Source: CAD feature listing. Evaluate the final solid. Frame: model axes, mm. A direction names the side the tool comes from. Give positions to 0.01 mm unless a question says otherwise; leave off trailing zeros. Loops run counter-clockwise (first coordinate to the right, second up) from the corner with the lowest first, then second, coordinate; pieces in that order, holes last. Notation, with made-up numbers: (-39.5, 88.5) - (-15.5, 88.5) arc R22 ccw to (-15.5, 121.5) - close; hole circle Ø11 at (-9.5, 45.5). An arc over 180 degrees is marked (long way). Put each result on its own line as item: value.
Autodesk Inventor part; units mm, degrees
ref_plane "YZ Plane" through (0, 0, 0) normal (1, 0, 0) x (0, 1, 0)
ref_plane "XZ Plane" through (0, 0, 0) normal (0, 1, 0) x (-1, 0, 0)
ref_plane "XY Plane" through (0, 0, 0) normal (0, 0, 1) x (1, 0, 0)
sketch "Sketch1" plane through (0, 0, 0) normal (0, 0, 1) x (1, 0, 0)
  line L0 (-4, 10) -> (-4, 14)
  line L1 (0, 10) -> (-4, 10)
  line L2 (0, 14) -> (0, 10) construction
  line L3 (0, 14) -> (-4, 14)
  line L4 (-4, -16) -> (-4, 0)
  line L5 (0, -16) -> (-4, -16)
  line L6 (0, 0) -> (0, -16) construction
  line L7 (0, 0) -> (-4, 0)
  line L8 (0, 6.5) -> (0, 3.5)
  line L9 (0, 6.5) -> (12, 6.5)
  line L10 (12, 6.5) -> (12, 3.5)
  line L11 (12, 3.5) -> (0, 3.5)
  line L12 (0, 3.5) -> (0, 6.5)
  line L13 (0, 10) -> (0, 6.5)
  line L14 (0, 3.5) -> (0, 0)
  line L15 (4.8, 7.7) -> (7.2, 7.7)
  line L16 (7.2, 7.7) -> (7.2, 2.3)
  line L17 (7.2, 2.3) -> (4.8, 2.3)
  line L18 (4.8, 2.3) -> (4.8, 7.7)
  line L19 (11.3, -2.5) -> (23.3, -2.5)
  line L20 (23.3, -2.5) -> (23.3, -5.5)
  line L21 (23.3, -5.5) -> (11.3, -5.5)
  line L22 (11.3, -5.5) -> (11.3, -2.5)
  line L23 (16.1, -1.3) -> (18.5, -1.3)
  line L24 (18.5, -1.3) -> (18.5, -6.7)
  line L25 (18.5, -6.7) -> (16.1, -6.7)
  line L26 (16.1, -6.7) -> (16.1, -1.3)
  line L27 (0, 14) -> (27.3, 14)
  line L28 (27.3, 14) -> (27.3, 4)
  line L29 (27.3, 4) -> (23.3, 4)
  line L30 (23.3, 4) -> (23.3, -12)
  line L31 (23.3, -12) -> (27.3, -12)
  line L32 (27.3, -12) -> (27.3, -16)
  line L33 (27.3, -16) -> (0, -16)
  point P0 (7.2, 5)
  point P1 (12, 5)
  point P2 (6, 7.7)
  point P3 (6, 6.5)
  point P4 (16.1, -4)
  point P5 (11.3, -4)
  point P6 (17.3, -1.3)
  point P7 (17.3, -2.5)
  point P8 (23.3, -4)
  point P9 (23.3, -4)
  point P10 (4.8, 6.5)
  point P11 (7.2, 6.5)
  point P12 (7.2, 3.5)
  point P13 (4.8, 3.5)
  point P14 (18.5, -5.5)
  point P15 (16.1, -5.5)
  point P16 (16.1, -2.5)
  point P17 (18.5, -2.5)
  dimension "d0" = 12
  dimension "d1" = 3
  dimension "d2" = 5.4
  dimension "d3" = 2.4
  dimension "d4" = 12
  dimension "d5" = 3
  dimension "d6" = 2.4
  dimension "d7" = 5.4
  dimension "d8" = 4
  dimension "d10" = 10
  dimension "d11" = 23.3
  dimension "d12" = 4
extrude "Extrusion1" add sketch "Sketch1" along normal blind 4 contours L0 L3 L27 L28 L29 L30 L19 L24 L23 L26 L22 L21 L25 L31 L32 L33 L5 L4 L7 L14 L11 L18 L17 L16 L10 L9 L15 L13 L1
properties part number "Door_LimitSwitch_Holder_Side_1" material "MDF Medium Density Fiberboard"
1) Access query for faces 4 (the flat face through (12, -16, 2)), 5 (the flat face through (2, 3.5, 2)), 6 (the flat face through (21, -2.5, 2)), 7 (the flat face through (16.1, -6, 2)). Directions: +Z, -Z, +X, -X, +Y, -Y. A direction counts if a zero-diameter tool reaches every point of the face in a straight line with its end or side. Return the directions, or none.
Check result:
face 4: +Z, -Z, +X, -X, -Y
face 5: +Z, -Z, -X
face 6: +Z, -Z, +X
face 7: +Z, -Z
2) Mould query, pull axis X, two halves, no side actions, for faces 1 (the flat face through (-4, 12, 2)), 2 (the flat face through (18.5, -6, 2)), 3 (the flat face through (11, 14, 2)). Classes: pulls with the +X half, pulls with the -X half, needs draft (parallel to the pull), parting line crosses it, or undercut.
Check result:
face 1: pulls with the -X half
face 2: undercut
face 3: needs draft
3) Section query C-C, the plane y = -8.25. Output: boundary loops of the cut face in (x, z), plus the area to 3 significant figures.
Check result:
outline: (-4, 0) - (23.3, 0) - (23.3, 4) - (-4, 4) - close
area: 109 mm²
4) Pin query (flat end, axial travel): P1, Ø1.3, axis at y = -2, z = 2, coming from the +X side; P2, Ø0.6, axis at y = 7, z = 1.5, coming from the -X side; P3, Ø0.9, axis at y = -3.5, z = 2.5, coming from the +X side. Return the tip coordinate at first contact, or that it passes through.
Check result:
P1: x = 23.3
P2: x = 0
P3: x = 11.3
5) Section query A-A, the plane x = 12.5. Output: boundary loops of the cut face in (y, z), plus the area to 3 significant figures.
Check result:
outline: (-16, 0) - (-5.5, 0) - (-5.5, 4) - (-16, 4) - close; (-2.5, 0) - (14, 0) - (14, 4) - (-2.5, 4) - close
area: 108 mm²
6) Section query B-B, the plane y = -1.75. Output: boundary loops of the cut face in (x, z), plus the area to 3 significant figures.
Check result:
outline: (-4, 0) - (16.1, 0) - (16.1, 4) - (-4, 4) - close; (18.5, 0) - (23.3, 0) - (23.3, 4) - (18.5, 4) - close
area: 99.6 mm²
7) Material intervals for line 1 along Y through (x, z) = (14.5, 1); line 2 along Y through (x, z) = (8, 0.8); line 3 along X through (y, z) = (3, 1.4), sorted ascending. Write a range as [from, to].
Check result:
line 1: [-16, -5.5], [-2.5, 14]
line 2: [-16, 3.5], [6.5, 14]
line 3: [0, 4.8], [7.2, 23.3]
